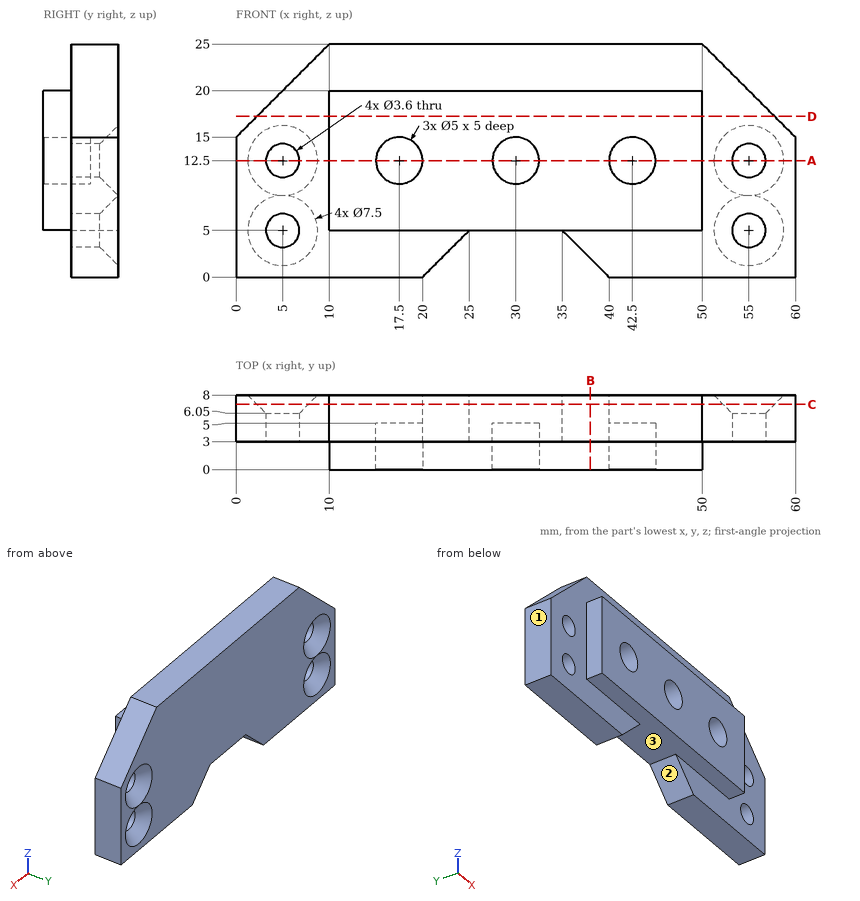
Here's the drawing with two shaded views (mm, measured from the low corner). I have some questions. A direction names the side the tool comes from. Give positions to 0.01 mm unless a question says otherwise; leave off trailing zeros. Loops run counter-clockwise (first coordinate to the right, second up) from the corner with the lowest first, then second, coordinate; pieces in that order, holes last. Notation, with made-up numbers: M 3.5,55 L 45.5,55 A18 ccw 45.5,70 Z; hole C 33.5,-37.5 d7. An arc over 180 degrees is marked long. Answer in a Markdown table with one row per item.
1. Suppose I cut it at B-B on x = 38. Write out the boundary of the cut face in (y, z).
Taken from the geometry:
| item | result |
|---|---|
| outline | M 0,5 L 3,5 L 3,2 L 8,2 L 8,25 L 3,25 L 3,20 L 0,20 Z |
2. If I drill on line 1 along Z through (x, y) = (55, 4.2); line 2 along Z through (x, y) = (42.5, 3.35); line 3 along X through (y, z) = (7.5, 10.5), over which ranges is the centre line in solid material (lowest first)?
Taken from the geometry:
| item | result |
|---|---|
| line 1 | z = 0 to 3.2, 6.8 to 10.7, 14.3 to 20 |
| line 2 | z = 0 to 10, 15 to 25 |
| line 3 | x = 0 to 2.44, 7.56 to 52.44, 57.56 to 60 |
3. Suppose I cut it at A-A on z = 12.5. Count the separate pieces of the cut face and the enclosed holes in it, plus the area to 3 significant figures.
Taken from the geometry:
| item | result |
|---|---|
| separate pieces | 3 |
| enclosed holes | 0 |
| area | 301 mm² |
4. Which directions (+Z, -Z, +X, -X, +Y, -Y) give clear straight access to the entire face, cutting with the end or side of a thin tool? Please do the marked faces 1, 2 and 3.
Taken from the geometry:
| item | result |
|---|---|
| face 1 | +Z, -Z, -X, +Y, -Y |
| face 2 | -Z, +Y, -Y |
| face 3 | -Z, -Y |
5. Suppose I cut it at D-D on z = 17.25. Write out the boundary of the cut face in (x, y).
Taken from the geometry:
| item | result |
|---|---|
| outline | M 2.25,3 L 10,3 L 10,0 L 50,0 L 50,3 L 57.75,3 L 57.75,8 L 2.25,8 Z |
6. For pin 1 Ø0.9 at (y, z) = (1, 9) entering from +X; pin 2 Ø4.5 at (x, z) = (5, 12.5) entering from +Y; pin 3 Ø4.5 at (x, z) = (42.5, 12.5) entering from -Y, each with a flat end and sliding along its axis, tell me the tip position at first contact or that it passes through.
Taken from the geometry:
| item | result |
|---|---|
| pin 1 | stops at x = 50 |
| pin 2 | stops at y = 6.5 |
| pin 3 | stops at y = 5 |
7. Suppose I cut it at C-C on y = 7. Write out the boundary of the cut face in (x, z).
Taken from the geometry:
| item | result |
|---|---|
| outline | M 0,0 L 20,0 L 25,5 L 35,5 L 40,0 L 60,0 L 60,15 L 50,25 L 10,25 L 0,15 Z; hole C 5,5 d5.5; hole C 5,12.5 d5.5; hole C 55,5 d5.5; hole C 55,12.5 d5.5 |
